```python
from build123d import *

# Parameters (mm, degrees)
SKETCH1_W                      = 260.35
SKETCH1_H                      = 190.5
BASE_DEPTH                     = 10.25
SKETCH2_R                      = 65
HOLES_DEPTH                    = 323.765293983
M8_ARM_MOUNT_HOLES_D           = 6.8
M8_ARM_MOUNT_HOLES_CSINK_D     = 10
M8_ARM_MOUNT_HOLES_CSINK_ANGLE = 90
FILLET1_R                      = 15.5


with BuildPart() as part:
    # Sketch1 → Base (new body)
    with BuildSketch(Plane(origin=(0, 0, 0), x_dir=(1, 0, 0), z_dir=(0, 1, 0))):
        with Locations((130.175, 95.25)):
            Rectangle(SKETCH1_W, SKETCH1_H)
    extrude(amount=BASE_DEPTH)

    # Sketch2 → Holes (cut, through all)
    with BuildSketch(Plane(origin=(0, 10.25, 0), x_dir=(1, 0, 0), z_dir=(0, 1, 0))):
        with Locations(Location((130.175, 95.25, 0), (0, 0, 270))):
            Circle(SKETCH2_R)
        with BuildLine():
            Line((206.35, 19), (226.35, 19))
            ThreePointArc((226.35, 19), (230.35, 15), (226.35, 11))
            Line((226.35, 11), (206.35, 11))
            ThreePointArc((206.35, 11), (202.35, 15), (206.35, 19))
        make_face()
        with BuildLine():
            Line((241.35, 15), (241.35, 35))
            ThreePointArc((241.35, 35), (245.35, 39), (249.35, 35))
            Line((249.35, 35), (249.35, 15))
            ThreePointArc((249.35, 15), (245.35, 11), (241.35, 15))
        make_face()
        with BuildLine():
            Line((11, 15), (11, 35))
            ThreePointArc((11, 35), (15, 39), (19, 35))
            Line((19, 35), (19, 15))
            ThreePointArc((19, 15), (15, 11), (11, 15))
        make_face()
        with BuildLine():
            Line((11, 155.5), (11, 175.5))
            ThreePointArc((11, 175.5), (15, 179.5), (19, 175.5))
            Line((19, 175.5), (19, 155.5))
            ThreePointArc((19, 155.5), (15, 151.5), (11, 155.5))
        make_face()
        with BuildLine():
            Line((241.35, 155.5), (241.35, 175.5))
            ThreePointArc((241.35, 175.5), (245.35, 179.5), (249.35, 175.5))
            Line((249.35, 175.5), (249.35, 155.5))
            ThreePointArc((249.35, 155.5), (245.35, 151.5), (241.35, 155.5))
        make_face()
        with BuildLine():
            Line((34, 19), (54, 19))
            ThreePointArc((54, 19), (58, 15), (54, 11))
            Line((54, 11), (34, 11))
            ThreePointArc((34, 11), (30, 15), (34, 19))
        make_face()
        with BuildLine():
            Line((206.35, 179.5), (226.35, 179.5))
            ThreePointArc((226.35, 179.5), (230.35, 175.5), (226.35, 171.5))
            Line((226.35, 171.5), (206.35, 171.5))
            ThreePointArc((206.35, 171.5), (202.35, 175.5), (206.35, 179.5))
        make_face()
        with BuildLine():
            Line((34, 179.5), (54, 179.5))
            ThreePointArc((54, 179.5), (58, 175.5), (54, 171.5))
            Line((54, 171.5), (34, 171.5))
            ThreePointArc((34, 171.5), (30, 175.5), (34, 179.5))
        make_face()
    extrude(amount=-HOLES_DEPTH, mode=Mode.SUBTRACT)

    # M8 Arm Mount Holes (through all)
    with Locations(Plane(origin=(0, 10.25, 0), x_dir=(1, 0, 0), z_dir=(0, 1, 0))):
        with Locations((70.175, 155.25), (190.175, 155.25), (190.175, 35.25), (70.175, 35.25)):
            CounterSinkHole(M8_ARM_MOUNT_HOLES_D / 2, M8_ARM_MOUNT_HOLES_CSINK_D / 2, counter_sink_angle=M8_ARM_MOUNT_HOLES_CSINK_ANGLE)

    # Fillet1
    fillet1_edges = [part.edges().sort_by_distance(p)[0] for p in [
        (0, 5.125, -190.5),
        (260.35, 5.125, -190.5),
        (260.35, 5.125, 0),
        (0, 5.125, 0),
    ]]
    fillet(fillet1_edges, radius=FILLET1_R)


solid = part.part
```
CAD build for the part. Positions are in the model's coordinates, mm. A direction names the side the tool comes from. Round coordinates to 2 decimals unless told otherwise and drop trailing zeros. Order: outer loops, then holes, each group sorted by start corner. A loop starts at its lowest first (then second) coordinate and runs counter-clockwise, first axis right, second up. Notation, with made-up numbers: (46.5, 73) - (55.5, 73) arc R27 cw to (55.5, 92) - close; hole circle Ø1 at (69, 20.5). An arc over 180 degrees is marked (long way). Answer in a Markdown table with one row per item. Add a question column.
(1) Band-saw the part on D-D on y = 6.5. Count the separate pieces of the cut face and the enclosed holes in it, and give its area (3 significant figures).
(2) Band-saw the part on A-A on z = -95.25. List the corners of the cut face in (x, y) (3 decimals), and give its area (3 significant figures).
(3) Band-saw the part on C-C on x = 107.5. List the corners of the cut face in (y, z).
(4) Mould opens along Z. For faces 1 (the face through (241.35, 5, -165)), 2 (the face through (260.35, 5, -94)), 3 (the face through (4.42, 5.2, -4.66)) say: +Z half, -Z half, draft (parallel to the pull), parting line (faces both ways), or undercut.
(5) Band-saw the part on B-B on x = 216. List the corners of the cut face in (y, z).
(6) 3-axis set-ups, long thin cutter, end or side, ignore diameter. For faces 4 (the face through (11, 5, -25)), 5 (the face through (4.42, 5.2, -185.84)): which of +Z, -Z, +X, -X, +Y, -Y reach the whole face in a straight line?
(7) Probe L1, parallel to X at y = 3.75, z = -97; L2, parallel to X at y = 3, z = -23.5; L3, parallel to X at y = 2, z = -12. List the from-to ranges inside material, lowest first. Write a range as [from, to].
Data:
| question | item | result |
|---|---|---|
| 1 | separate pieces | 1 |
| 1 | enclosed holes | 13 |
| 1 | area | 34,300 mm^2 |
| 2 | outline | (0, 0) - (65.175, 0) - (65.175, 10.25) - (0, 10.25) - close; (195.175, 0) - (260.35, 0) - (260.35, 10.25) - (195.175, 10.25) - close |
| 2 | area | 1,340 mm^2 |
| 3 | outline | (0, -190.5) - (10.25, -190.5) - (10.25, -156.17) - (0, -156.17) - close; (0, -34.33) - (10.25, -34.33) - (10.25, 0) - (0, 0) - close |
| 4 | face 1 | undercut |
| 4 | face 2 | draft |
| 4 | face 3 | +Z half |
| 5 | outline | (0, -190.5) - (10.25, -190.5) - (10.25, -179.5) - (0, -179.5) - close; (0, -171.5) - (10.25, -171.5) - (10.25, -19) - (0, -19) - close; (0, -11) - (10.25, -11) - (10.25, 0) - (0, 0) - close |
| 6 | face 4 | +Y, -Y |
| 6 | face 5 | -Z, -X, +Y, -Y |
| 7 | L1 | x = [0, 65.2], [195.15, 260.35] |
| 7 | L2 | x = [0, 11], [19, 241.35], [249.35, 260.35] |
| 7 | L3 | x = [0.4, 12.35], [17.65, 31.35], [56.65, 203.7], [229, 242.7], [248, 259.95] |
